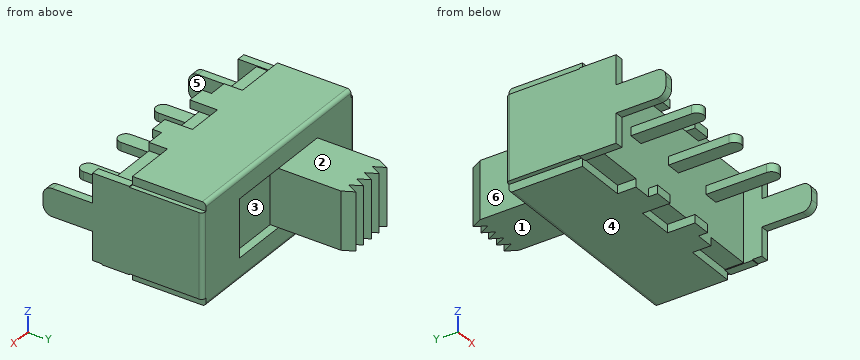
```python
from build123d import *

# Parameters (mm, degrees)
SKETCH_1_W          = 11.2
SKETCH_1_H          = 4.6
EXTRUDE_1_DEPTH     = 5
EXTRUDE_2_DEPTH     = 0.45
EXTRUDE_3_DEPTH     = 0.45
EXTRUDE_4_DEPTH     = 0.45
EXTRUDE_START       = 0.45
EXTRUDE_5_DEPTH     = 0.45
CUT_EXTRUDE_1_DEPTH = 0.45
SKETCH_7_W          = 3.12
SKETCH_7_H          = 3.15
EXTRUDE_6_DEPTH     = 4.45
CUT_EXTRUDE_2_DEPTH = 4.45
EXTRUDE_7_DEPTH     = 3.7
CUT_EXTRUDE_3_DEPTH = 3.7
FILLET_1_R          = 0.2
FILLET_2_R          = 0.2
FILLET_3_R          = 0.2
FILLET_4_R          = 0.2


with BuildPart() as part:
    # 草图1 → 凸台-拉伸1 (new body)
    with BuildSketch(Plane(origin=(0, 0, 0), x_dir=(1, 0, 0), z_dir=(0, 1, 0))):
        with Locations((5.6, 2.3)):
            Rectangle(SKETCH_1_W, SKETCH_1_H)
    extrude(amount=EXTRUDE_1_DEPTH)

    # 草图2 → 凸台-拉伸2 (add)
    with BuildSketch(Plane.XY):
        Polygon((11.4, 5), (11.4, 1), (8.6, 1), (8.6, 0), (7.6, 0), (7.6, -0.5), (6.6, -0.5), (6.6, 1), (5.6, 1), (4.6, 1), (4.6, -0.5), (3.6, -0.5), (3.6, 0), (2.6, 0), (2.6, 1), (-0.2, 1), (-0.2, 5), align=None)
    extrude(amount=EXTRUDE_2_DEPTH)

    # 草图3 → 凸台-拉伸3 (add)
    with BuildSketch(Plane(origin=(0, 0, -4.6), x_dir=(-1, 0, 0), z_dir=(0, 0, -1))):
        Polygon((-5.6, 5), (-11.4, 5), (-11.4, 1), (-8.6, 1), (-8.6, 0), (-7.6, 0), (-7.6, -0.5), (-6.6, -0.5), (-6.6, 1), (-4.6, 1), (-4.6, -0.5), (-3.6, -0.5), (-3.6, 0), (-2.6, 0), (-2.6, 1), (0.2, 1), (0.2, 5), align=None)
    extrude(amount=EXTRUDE_3_DEPTH)

    # 草图4 → 凸台-拉伸4 (add)
    with BuildSketch(Plane(origin=(11.2, 0, 0), x_dir=(0, 0, -1), z_dir=(1, 0, 0))):
        with BuildLine():
            Line((0, 5), (0, 1))
            Line((0, 1), (-0.05, 1))
            Line((-0.05, 1), (-0.05, -1))
            Line((-0.05, -1), (0, -1))
            Line((0, -1), (1.55, -1))
            Line((1.55, -1), (1.55, -3.2))
            ThreePointArc((1.55, -3.2), (1.696446609, -3.553553391), (2.05, -3.7))
            Line((2.05, -3.7), (2.3, -3.7))
            Line((2.3, -3.7), (2.55, -3.7))
            ThreePointArc((2.55, -3.7), (2.903553391, -3.553553391), (3.05, -3.2))
            Line((3.05, -3.2), (3.05, -1))
            Line((3.05, -1), (4.6, -1))
            Line((4.6, -1), (4.6, -0.5))
            Line((4.6, -0.5), (4.65, -0.5))
            Line((4.65, -0.5), (4.65, 1))
            Line((4.65, 1), (4.6, 1))
            Line((4.6, 1), (4.6, 5))
            Line((4.6, 5), (0, 5))
        make_face()
    extrude(amount=EXTRUDE_4_DEPTH)

    # 草图5 → 凸台-拉伸5 (add)
    with BuildSketch(Plane.ZY.offset(EXTRUDE_START)):
        with BuildLine():
            Line((-4.6, 5), (-4.6, 1))
            Line((-4.6, 1), (-4.65, 1))
            Line((-4.65, 1), (-4.65, -1))
            Line((-4.65, -1), (-4.6, -1))
            Line((-4.6, -1), (-3.05, -1))
            Line((-3.05, -1), (-3.05, -3.2))
            ThreePointArc((-3.05, -3.2), (-2.903553391, -3.553553391), (-2.55, -3.7))
            Line((-2.55, -3.7), (-2.05, -3.7))
            ThreePointArc((-2.05, -3.7), (-1.696446609, -3.553553391), (-1.55, -3.2))
            Line((-1.55, -3.2), (-1.55, -1))
            Line((-1.55, -1), (0.05, -1))
            Line((0.05, -1), (0.05, 1))
            Line((0.05, 1), (0, 1))
            Line((0, 1), (0, 5))
            Line((0, 5), (-4.6, 5))
        make_face()
    extrude(amount=-EXTRUDE_5_DEPTH)

    # 草图6 → 切除-拉伸1 (cut)
    with BuildSketch(Plane(origin=(0, 5, 0), x_dir=(1, 0, 0), z_dir=(0, 1, 0))):
        Polygon((2.48, 2.3), (2.48, 3.875), (8.72, 3.875), (8.72, 0.725), (2.48, 0.725), align=None)
    extrude(amount=-CUT_EXTRUDE_1_DEPTH, mode=Mode.SUBTRACT)

    # 草图7 → 凸台-拉伸6 (add)
    with BuildSketch(Plane(origin=(0, 4.55, 0), x_dir=(1, 0, 0), z_dir=(0, 1, 0))):
        with Locations((4.04, 2.3)):
            Rectangle(SKETCH_7_W, SKETCH_7_H)
    extrude(amount=EXTRUDE_6_DEPTH)

    # 草图8 → 切除-拉伸2 (cut)
    with BuildSketch(Plane.XY.offset(-0.725)):
        Polygon((2.48, 8.4), (2.792, 9), (2.48, 9), align=None)
        Polygon((3.104, 8.4), (3.416, 9), (2.792, 9), align=None)
        Polygon((3.728, 8.4), (4.04, 9), (3.416, 9), align=None)
        Polygon((4.352, 8.4), (4.664, 9), (4.04, 9), align=None)
        Polygon((5.288, 9), (4.664, 9), (4.976, 8.4), align=None)
        Polygon((5.6, 9), (5.288, 9), (5.6, 8.4), align=None)
    extrude(amount=-CUT_EXTRUDE_2_DEPTH, mode=Mode.SUBTRACT)

    # 草图9 → 凸台-拉伸7 (add)
    with BuildSketch(Plane.XZ):
        Polygon((8.2, -2.3), (8.2, -2.07), (9, -2.07), (9, -2.3), (9, -2.53), (8.2, -2.53), align=None)
        Polygon((5.2, -2.3), (5.2, -2.07), (6, -2.07), (6, -2.3), (6, -2.53), (5.2, -2.53), align=None)
        Polygon((2.2, -2.3), (2.2, -2.07), (3, -2.07), (3, -2.3), (3, -2.53), (2.2, -2.53), align=None)
    extrude(amount=EXTRUDE_7_DEPTH)

    # 草图10 → 切除-拉伸3 (cut)
    with BuildSketch(Plane.XY.offset(-2.07)):
        with BuildLine():
            ThreePointArc((2.6, -3.7), (2.317157288, -3.582842712), (2.2, -3.3))
            Line((2.2, -3.3), (2.2, -3.7))
            Line((2.2, -3.7), (2.6, -3.7))
        make_face()
        with BuildLine():
            ThreePointArc((3, -3.3), (2.882842712, -3.582842712), (2.6, -3.7))
            Line((2.6, -3.7), (3, -3.7))
            Line((3, -3.7), (3, -3.3))
        make_face()
        with BuildLine():
            Line((3, -3.3), (3, -3.7))
            Line((3, -3.7), (5.6, -3.7))
            ThreePointArc((5.6, -3.7), (5.317157288, -3.582842712), (5.2, -3.3))
            Line((5.2, -3.3), (3, -3.3))
        make_face()
        with BuildLine():
            ThreePointArc((6, -3.3), (5.882842712, -3.582842712), (5.6, -3.7))
            Line((5.6, -3.7), (8.6, -3.7))
            ThreePointArc((8.6, -3.7), (8.317157288, -3.582842712), (8.2, -3.3))
            Line((8.2, -3.3), (6, -3.3))
        make_face()
        with BuildLine():
            ThreePointArc((9, -3.3), (8.882842712, -3.582842712), (8.6, -3.7))
            Line((8.6, -3.7), (9, -3.7))
            Line((9, -3.7), (9, -3.3))
        make_face()
    extrude(amount=-CUT_EXTRUDE_3_DEPTH, mode=Mode.SUBTRACT)

    # 圆角1
    fillet_1_edges = [part.edges().sort_by_distance(p)[0] for p in [
        (-0.45, 5, -2.3),
    ]]
    fillet(fillet_1_edges, radius=FILLET_1_R)

    # 圆角2
    fillet_2_edges = [part.edges().sort_by_distance(p)[0] for p in [
        (5.6, 5, 0.45),
    ]]
    fillet(fillet_2_edges, radius=FILLET_2_R)

    # 圆角3
    fillet_3_edges = [part.edges().sort_by_distance(p)[0] for p in [
        (11.65, 5, -2.3),
    ]]
    fillet(fillet_3_edges, radius=FILLET_3_R)

    # 圆角4
    fillet_4_edges = [part.edges().sort_by_distance(p)[0] for p in [
        (5.6, 5, -5.05),
    ]]
    fillet(fillet_4_edges, radius=FILLET_4_R)


solid = part.part
```
CAD build for the part. Positions are in the model's coordinates, mm. Face numbers are marked on the shaded views. A direction names the side the tool comes from. Coordinates: 2 decimals unless noted, no trailing zeros. Order: outer loops, then holes, each group sorted by start corner. A loop starts at its lowest first (then second) coordinate and runs counter-clockwise, first axis right, second up.
(1) Saw through at D-D, the plane y = 0.5. Write the cut outline in (x, z).
Solution:
outline: (-0.45, -4.65) - (0, -4.65) - (0, -4.6) - (2.6, -4.6) - (2.6, -5.05) - (4.6, -5.05) - (4.6, -4.6) - (6.6, -4.6) - (6.6, -5.05) - (8.6, -5.05) - (8.6, -4.6) - (11.2, -4.6) - (11.2, -4.65) - (11.65, -4.65) - (11.65, 0.05) - (11.2, 0.05) - (11.2, 0) - (8.6, 0) - (8.6, 0.45) - (6.6, 0.45) - (6.6, 0) - (4.6, 0) - (4.6, 0.45) - (2.6, 0.45) - (2.6, 0) - (0, 0) - (0, 0.05) - (-0.45, 0.05) - close
(2) Which spindle directions (+Z, -Z, +X, -X, +Y, -Y) get a long thin tool onto all of the face, cutting with end or side? Do the marked faces 1, 2 and 3. Say none if no direction does.
Solution:
face 1: -Z, +X, -X, +Y
face 2: +Z, +X, -X, +Y
face 3: +Y
(3) Saw through at A-A, the plane y = -2.5. Write the cut outline in (x, z), and give its area (3 significant figures).
Solution:
outline: (-0.45, -3.05) - (0, -3.05) - (0, -1.55) - (-0.45, -1.55) - close; (2.2, -2.53) - (3, -2.53) - (3, -2.07) - (2.2, -2.07) - close; (5.2, -2.53) - (6, -2.53) - (6, -2.07) - (5.2, -2.07) - close; (8.2, -2.53) - (9, -2.53) - (9, -2.07) - (8.2, -2.07) - close; (11.2, -3.05) - (11.65, -3.05) - (11.65, -1.55) - (11.2, -1.55) - close
area: 2.45 mm2
(4) Drill centre lines: L1, parallel to X at y = -1, z = -2.6; L2, parallel to Y at x = 7.75, z = -4; L3, parallel to Y at x = 7.25, z = -1.9. Where is each one in solid material? Low to high.
Solution:
L1: x = -0.45 to 0, 11.2 to 11.65
L2: y = 0 to 5
L3: y = 0 to 4.55
(5) Saw through at C-C, the plane x = 8. Write the cut outline in (y, z) (3 decimals), and give its area (3 significant figures).
Solution:
outline: (0, -5.05) - (4.8, -5.05) arc R0.2 ccw to (5, -4.85) - (5, -3.875) - (4.55, -3.875) - (4.55, -0.725) - (5, -0.725) - (5, 0.25) arc R0.2 ccw to (4.8, 0.45) - (0, 0.45) - close
area: 26.1 mm2
(6) Pin check, flat tips, straight feed: pin 1 Ø1.5 at (y, z) = (7, -2.5) entering from -X; pin 2 Ø0.6 at (x, y) = (8.5, -2) entering from +Z. Stop position of each tip, or through.
Solution:
pin 1: stops at x = 2.48
pin 2: stops at z = -2.07
(7) Mould opens along X. For the marked faces 4, 5 and 6 say: released by +X, released by -X, zero draft, split by the parting line, or undercut.
Solution:
face 4: zero draft
face 5: undercut
face 6: released by -X
(8) Saw through at B-B, the plane z = -3.25. Write the cut outline in (x, y), and give its area (3 significant figures).
Solution:
outline: (-0.45, -1) - (0, -1) - (0, 0) - (11.2, 0) - (11.2, -1) - (11.65, -1) - (11.65, 4.8) arc R0.2 ccw to (11.45, 5) - (8.72, 5) - (8.72, 4.55) - (5.6, 4.55) - (5.6, 8.4) - (5.29, 9) - (4.98, 8.4) - (4.66, 9) - (4.35, 8.4) - (4.04, 9) - (3.73, 8.4) - (3.42, 9) - (3.1, 8.4) - (2.79, 9) - (2.48, 8.4) - (2.48, 5) - (-0.25, 5) arc R0.2 ccw to (-0.45, 4.8) - close
area: 71.5 mm2
